Geometry check sheet. Reference: the model listing, model coordinates, mm. Coordinates: 2 decimals unless noted, no trailing zeros. Write each loop counter-clockwise with the first axis right and the second up, starting at its lowest first coordinate (ties: lowest second). Pieces come first, ordered by that corner, then holes.
from build123d import *

# Parameters (mm, degrees)
POCKET008003002_DEPTH = 5


with BuildPart() as obj1:
    # Sketch024 → Revolution001 (revolve)
    with BuildSketch(Plane.XZ):
        Polygon((0, 0), (0, -60), (1.5, -58.5), (1.5, 0), align=None)
    revolve(axis=Axis((0, 0, 0), (1, 0, 0)))


with BuildPart() as slidergroove:
    # Part__Mirroring006: instance of obj1
    add(obj1.part.mirror(Plane(origin=(0, 0, 0), x_dir=(0, -1, 0), z_dir=(1, 0, 0))))

    # Fusion: union obj1
    add(obj1.part)

    # Sketch025 → Pocket008003002 (cut)
    with BuildSketch(Plane(origin=(-1.5, 0, 0), x_dir=(0, -1, 0), z_dir=(-1, 0, 0))):
        Polygon((-100, 100), (100, 100), (100, -58), (-5, -58), (-5, -66), (-100, -66), align=None)
    extrude(amount=-POCKET008003002_DEPTH, mode=Mode.SUBTRACT)


solid = slidergroove.part
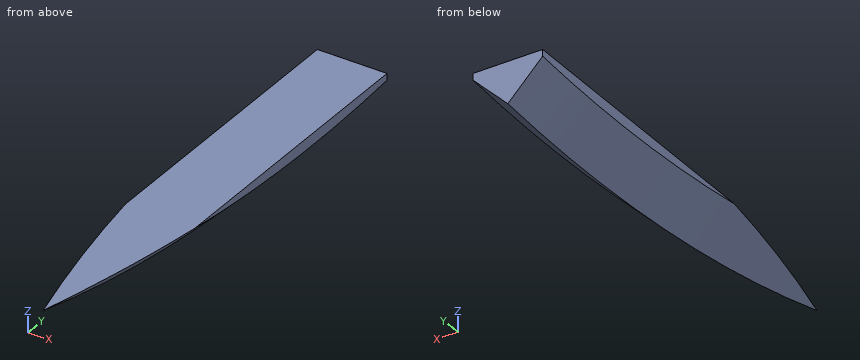
1. Sectioned sample at A-A, the plane x = 0.3. Record the boundary of the cut face in (y, z), and give its area (3 significant figures).
Computed values:
outline: (-14.15, -58) arc R59.7 ccw to (5, -59.49) - (5, -58) - close
area: 24.2 mm2
2. Sectioned sample at B-B, the plane x = -0.65. Record the boundary of the cut face in (y, z), and give its area (3 significant figures).
Computed values:
outline: (-12.59, -58) arc R59.35 ccw to (5, -59.14) - (5, -58) - close
area: 17.8 mm2
3. Thickness scan on line 1 along Z through (x, y) = (-0.6, -5); line 2 along Z through (x, y) = (-1, -8.5); line 3 along X through (y, z) = (-14, -58.25). Record the ranges inside material, lowest first.
Computed values:
line 1: z = -59.19 to -58
line 2: z = -58.38 to -58
line 3: x = -0.09 to 0.09
